```python
from build123d import *

# Parameters (mm, degrees)
F0_W     = 43
F0_H     = 264
F1_DEPTH = 10.5


with BuildPart() as f1:
    # F0 (on Front) → F1 (new body)
    with BuildSketch(Plane.XZ):
        Polygon((275, 155), (275, 175), (-275, 175), (-275, 155), (-295, 155), (-295, 132), (-252, 132), (252, 132), (295, 132), (295, 155), align=None)
        with Locations((273.5, 0)):
            Rectangle(F0_W, F0_H)
        with Locations((-273.5, 0)):
            Rectangle(F0_W, F0_H)
        Polygon((295, -155), (295, -132), (252, -132), (-252, -132), (-295, -132), (-295, -155), (-275, -155), (-275, -175), (275, -175), (275, -155), align=None)
    extrude(amount=F1_DEPTH)


solid = f1.part
```
Input: part model. Units: mm. Frame: model coordinates. A direction names the side the tool comes from. Round coordinates to 2 decimals unless told otherwise and drop trailing zeros. Write each loop counter-clockwise with the first axis right and the second up, starting at its lowest first coordinate (ties: lowest second). Pieces come first, ordered by that corner, then holes. Notation, with made-up numbers: M 43,72 L 83,72 A11 cw 83,77 Z; hole C -39.75,30.5 d3. An arc over 180 degrees is marked long. Write each question's results on one line, items separated by ' | '.
Q1. Line query: line 1 along Z through (x, y) = (143, -2.75); line 2 along X through (y, z) = (-8.75, -118.5). Output: solid intervals per line, ascending.
Results:
line 1: z = -175 to -132, 132 to 175 | line 2: x = -295 to -252, 252 to 295
Q2. Section query C-C (x = 137.5). Return loops of the section in (y, z), and give its area (3 significant figures).
Results:
outline: M -10.5,-175 L 0,-175 L 0,-132 L -10.5,-132 Z; M -10.5,132 L 0,132 L 0,175 L -10.5,175 Z | area: 903 mm^2
Q3. Access query for faces 4 (the face through (-285, -5, 155)), 5 (the face through (285, -5, -155)), 6 (the face through (252, -5, -2)), 7 (the face through (-285, -5, -155)). Directions: +Z, -Z, +X, -X, +Y, -Y. A direction counts if a zero-diameter tool reaches every point of the face in a straight line with its end or side. Return the directions, or none.
Results:
face 4: +Z, -X, +Y, -Y | face 5: -Z, +X, +Y, -Y | face 6: +Y, -Y | face 7: -Z, -X, +Y, -Y
Q4. Section query B-B (z = -55). Return loops of the section in (x, y), and give its area (3 significant figures).
Results:
outline: M -295,-10.5 L -252,-10.5 L -252,0 L -295,0 Z; M 252,-10.5 L 295,-10.5 L 295,0 L 252,0 Z | area: 903 mm^2
Q5. Section query A-A (y = -6.5). Return loops of the section in (x, z).
Results:
outline: M -295,-155 L -275,-155 L -275,-175 L 275,-175 L 275,-155 L 295,-155 L 295,155 L 275,155 L 275,175 L -275,175 L -275,155 L -295,155 Z; hole M -252,-132 L 252,-132 L 252,132 L -252,132 Z
Q6. Pin query (flat end, axial travel): P1, Ø3, axis at y = -5.5, z = -167.5, coming from the -X side; P2, Ø3, axis at y = -6.5, z = 169, coming from the +X side; P3, Ø5, axis at x = -289, y = -3.5, coming from the +Z side. Return the tip coordinate at first contact, or that it passes through.
Results:
P1: stops at x = -275 | P2: stops at x = 275 | P3: stops at z = 155
Q7. Draft query along X for faces 1 (the face through (-4, -5, 132)), 2 (the face through (-295, -5, 2)), 3 (the face through (4, -5, 175)). Return one class per face: released by +X, released by -X, zero draft, split by the parting line, or undercut.
Results:
face 1: undercut | face 2: released by -X | face 3: zero draft
